Here's how the part is built. I have some questions about the finished solid (model axes, mm). A direction names the side the tool comes from. Give positions to 0.01 mm unless a question says otherwise; leave off trailing zeros. Loops run counter-clockwise (first coordinate to the right, second up) from the corner with the lowest first, then second, coordinate; pieces in that order, holes last.
Q1. Suppose I cut it at A-A (z = 0). List the corners of the cut face in (x, y) for me.
Q2. Suppose I cut it at C-C (x = 71.12). List the corners of the cut face in (y, z) for me, and give its area (3 significant figures).
Q3. I'm going to push flat-ended pins straight in: P1, Ø8.5, axis at x = 72.82, z = 50.99, coming from the +Y side; P2, Ø15, axis at x = 81.63, z = -35.21, coming from the +Y side; P3, Ø2, axis at x = 80, y = 1, coming from the +Z side; P4, Ø1.5, axis at y = 1.5, z = -39.5, coming from the -X side. Where does each tip first touch, or does it pass through?
Q4. Suppose I cut it at B-B (y = 2). Count the separate pieces of the cut face and the enclosed holes in it, and give its area (3 significant figures).
Q5. For faces 5 (the face through (71.783, 3.131, 18.895)), 6 (the face through (68.003, 3.131, -34.381)), 7 (the face through (35.49, 3.13, -18.49)), which set-ups out of +Z, -Z, +X, -X, +Y, -Y let a thin tool reach every point of the face, with its end or its side?
Q6. Suppose I cut it at D-D (x = 88.9). List the corners of the cut face in (y, z) for me, and give its area (3 significant figures).
Q7. Thinking about a two-plate mould opening in X: for faces 1 (the face through (66, 0, -1)), 2 (the face through (65.31, 3.13, 61.23)), 3 (the face through (44.534, 3.131, 15.621)), 4 (the face through (68.142, 3.131, 34.105)), which applies, pulls with the +X half, pulls with the -X half, needs draft (parallel to the pull), parting line crosses it, or undercut?
Q8. I need wall thicknesses on probe 1 along X at (y, z) = (4.5, 0.5); probe 2 along Z at (x, y) = (78, 2.5); probe 3 along Z at (x, y) = (67, 6). Which ranges of each line are inside material? Lowest first, please.
```python
from build123d import *

# Parameters (mm, degrees)
SKETCH1_R           = 2.0828
SKETCH1_R_2         = 4.6736
BOSS_EXTRUDE1_DEPTH = 6.35


with BuildPart() as part:
    # Sketch1 → Boss-Extrude1 (new body)
    with BuildSketch(Plane(origin=(0, 0, 0), x_dir=(1, 0, 0), z_dir=(0, 1, 0))):
        with BuildLine():
            Line((67.725064599, 15.875), (52.484642113, 12.302589868))
            ThreePointArc((52.484642113, 12.302589868), (49.586387593, 12.302563925), (46.99, 13.590450074))
            Line((46.99, 13.590450074), (42.145459513, 17.594564059))
            ThreePointArc((42.145459513, 17.594564059), (35.395020139, 18.445048647), (31.75, 12.7))
            Line((31.75, 12.7), (31.75, -12.7))
            ThreePointArc((31.75, -12.7), (35.395020139, -18.445048647), (42.145459513, -17.594564059))
            Line((42.145459513, -17.594564059), (46.99, -13.590450074))
            ThreePointArc((46.99, -13.590450074), (49.586387593, -12.302563925), (52.484642113, -12.302589868))
            Line((52.484642113, -12.302589868), (67.725064599, -15.875))
            ThreePointArc((67.725064599, -15.875), (71.818943633, -18.959526957), (72.300962181, -24.062644653))
            ThreePointArc((72.300962181, -24.062644653), (68.072487407, -34.242903765), (62.419385775, -43.70652445))
            ThreePointArc((62.419385775, -43.70652445), (65.538195996, -61.394176154), (83.2258477, -58.275365933))
            ThreePointArc((83.2258477, -58.275365933), (101.6, 0), (83.2258477, 58.275365933))
            ThreePointArc((83.2258477, 58.275365933), (65.538195996, 61.394176154), (62.419385775, 43.70652445))
            ThreePointArc((62.419385775, 43.70652445), (68.072487407, 34.242903765), (72.300962181, 24.062644653))
            ThreePointArc((72.300962181, 24.062644653), (71.818943633, 18.959526957), (67.725064599, 15.875))
        make_face()
        with Locations(Location((38.1, 12.7, 0), (0, 0, 270))):
            Circle(SKETCH1_R, mode=Mode.SUBTRACT)
        with Locations(Location((88.9, 0, 0), (0, 0, 270))):
            Circle(SKETCH1_R_2, mode=Mode.SUBTRACT)
        with Locations(Location((87.063381275, -17.97714218, 0), (0, 0, 270))):
            Circle(SKETCH1_R_2, mode=Mode.SUBTRACT)
        with Locations(Location((81.629411902, -35.211491201, 0), (0, 0, 270))):
            Circle(SKETCH1_R_2, mode=Mode.SUBTRACT)
        with Locations(Location((72.822616737, -50.990945192, 0), (0, 0, 270))):
            Circle(SKETCH1_R_2, mode=Mode.SUBTRACT)
        with Locations(Location((87.063381275, 17.97714218, 0), (0, 0, 270))):
            Circle(SKETCH1_R_2, mode=Mode.SUBTRACT)
        with Locations(Location((81.629411902, 35.211491201, 0), (0, 0, 270))):
            Circle(SKETCH1_R_2, mode=Mode.SUBTRACT)
        with Locations(Location((72.822616737, 50.990945192, 0), (0, 0, 270))):
            Circle(SKETCH1_R_2, mode=Mode.SUBTRACT)
        with Locations(Location((71.12, 0, 0), (0, 0, 270))):
            Circle(SKETCH1_R_2, mode=Mode.SUBTRACT)
        with Locations(Location((53.34, 0, 0), (0, 0, 270))):
            Circle(SKETCH1_R_2, mode=Mode.SUBTRACT)
        with Locations(Location((38.1, -12.7, 0), (0, 0, 90))):
            Circle(SKETCH1_R, mode=Mode.SUBTRACT)
    extrude(amount=BOSS_EXTRUDE1_DEPTH)


solid = part.part
```
Solutions:
1. outline: (31.75, 0) - (48.67, 0) - (48.67, 6.35) - (31.75, 6.35) - close; (58.01, 0) - (66.45, 0) - (66.45, 6.35) - (58.01, 6.35) - close; (75.79, 0) - (84.23, 0) - (84.23, 6.35) - (75.79, 6.35) - close; (93.57, 0) - (101.6, 0) - (101.6, 6.35) - (93.57, 6.35) - close
2. outline: (0, -63.58) - (6.35, -63.58) - (6.35, -55.34) - (0, -55.34) - close; (0, -46.64) - (6.35, -46.64) - (6.35, -27.36) - (0, -27.36) - close; (0, -17.95) - (6.35, -17.95) - (6.35, -4.67) - (0, -4.67) - close; (0, 4.67) - (6.35, 4.67) - (6.35, 17.95) - (0, 17.95) - close; (0, 27.36) - (6.35, 27.36) - (6.35, 46.64) - (0, 46.64) - close; (0, 55.34) - (6.35, 55.34) - (6.35, 63.58) - (0, 63.58) - close
2. area: 518 mm2
3. P1: passes through
3. P2: stops at y = 6.35
3. P3: stops at z = 62.09
3. P4: stops at x = 64.7
4. separate pieces: 1
4. enclosed holes: 11
4. area: 4,000 mm2
5. face 5: +Y, -Y
5. face 6: -X, +Y, -Y
5. face 7: -Z, +Y, -Y
6. outline: (0, -49.19) - (6.35, -49.19) - (6.35, -22.27) - (0, -22.27) - close; (0, -13.68) - (6.35, -13.68) - (6.35, -4.67) - (0, -4.67) - close; (0, 4.67) - (6.35, 4.67) - (6.35, 13.68) - (0, 13.68) - close; (0, 22.27) - (6.35, 22.27) - (6.35, 49.19) - (0, 49.19) - close
6. area: 456 mm2
7. face 1: needs draft
7. face 2: parting line crosses it
7. face 3: undercut
7. face 4: pulls with the -X half
8. probe 1: x = 31.75 to 48.69, 57.99 to 66.47, 75.77 to 84.25, 93.55 to 101.6
8. probe 2: z = -62.59 to -38.16, -32.27 to 32.27, 38.16 to 62.59
8. probe 3: z = -62.28 to -36.3, -15.71 to -2.21, 2.21 to 15.71, 36.3 to 62.28
